Read the model definition and answer for the solid it produces. Units are mm, in the model's axes. A direction names the side the tool comes from. Give positions to 0.01 mm unless a question says otherwise; leave off trailing zeros. Loops run counter-clockwise (first coordinate to the right, second up) from the corner with the lowest first, then second, coordinate; pieces in that order, holes last.
(1) Which of the six approach directions +Z, -Z, +X, -X, +Y, -Y give full straight-line access (tool end or side, diameter ignored) to faces 4 (the face through (-2, 0, 0)), 5 (the face through (0, 0, 3)), 6 (the face through (2.44, -0.54, 5.8))?
(2) Find section B-B, the plane z = 9. Write down the section's boundary in (x, y), then the cut area to 3 significant figures.
(3) Determine the mould class of faces 1 (the face through (0, 0, 10)), 2 (the face through (5.37, -1.19, 1.01)), 3 (the face through (0.74, -1.305, 1.479)) for opening direction Y: pulls with the +Y half, pulls with the -Y half, needs draft (parallel to the pull), parting line crosses it, or undercut.
(4) Find section A-A, the plane y = 0. Write down the section's boundary in (x, z).
(5) Straight lines are drawn through the part: probe 1 along Z at (x, y) = (-3.5, -1.25); probe 2 along Y at (x, z) = (1, 1.5); probe 3 along Y at (x, z) = (0.25, 0.75). For each, find the intervals that lie inside material, in ascending order.
(6) Each of these flat-tipped pins is pushed along its axis until it touches: P1, Ø2, axis at x = -1.5, z = 7.5, coming from the -Y side; P2, Ø1.5, axis at x = -0.5, y = 0, coming from the -Z side; P3, Ø2, axis at y = 0.5, z = 7, coming from the -X side. Where does it stop, or does it pass through?
Autodesk Inventor part; units mm, degrees
ref_plane "YZ Plane" through (0, 0, 0) normal (1, 0, 0) x (0, 1, 0)
ref_plane "XZ Plane" through (0, 0, 0) normal (0, 1, 0) x (-1, 0, 0)
ref_plane "XY Plane" through (0, 0, 0) normal (0, 0, 1) x (1, 0, 0)
sketch "Sketch1" plane through (0, 0, 0) normal (1, 0, 0) x (0, 1, 0)
  line L0 (0, 0) -> (5.5, 0)
  line L1 (5.5, 0) -> (5.5, 2)
  line L2 (5.5, 2) -> (2.5, 2)
  line L3 (2.5, 2) -> (2.5, 10)
  line L4 (2.5, 10) -> (0, 10)
  line L5 (0, 10) -> (0, 0)
  dimension "d0" = 8
  dimension "d1" = 2
  dimension "d2" = 5.5
  dimension "d3" = 2.5
revolve "Revolution1" add sketch "Sketch1" angle 360 about axis through (0, 0, 10) along (0, 0, -1)
fillet "Fillet1" radius 0.5 3 edges at (0, -5.5, 0) (0, -5.5, 2) (0, -2.5, 10)
sketch "Sketch2" plane through (0, 0, 0) normal (0, 0, -1) x (-1, 0, 0)
  circle A0 centre (0, 0) radius 5
  line L0 (1.5, -0.866) -> (0, -1.7321)
  line L1 (0, -1.7321) -> (-1.5, -0.866)
  line L2 (-1.5, -0.866) -> (-1.5, 0.866)
  line L3 (-1.5, 0.866) -> (0, 1.7321)
  line L4 (0, 1.7321) -> (1.5, 0.866)
  line L5 (1.5, 0.866) -> (1.5, -0.866)
  dimension "d6" = 3
extrude "Extrusion1" cut sketch "Sketch2" against normal blind 3 contours L0 L1 L2 L3 L4 L5
thread "Thread1"
properties part number "M5x8 low profile screw"
Entries:
1. face 4: -Z, +X, -X, +Y, -Y
1. face 5: -Z
1. face 6: +Z
2. outline: circle Ø5 at (0, 0)
2. area: 19.6 mm2
3. face 1: needs draft
3. face 2: parting line crosses it
3. face 3: undercut
4. outline: (-5.5, 0.5) arc R0.5 ccw to (-5, 0) - (-1.5, 0) - (-1.5, 3) - (1.5, 3) - (1.5, 0) - (5, 0) arc R0.5 ccw to (5.5, 0.5) - (5.5, 1.5) arc R0.5 ccw to (5, 2) - (2.5, 2) - (2.5, 9.5) arc R0.5 ccw to (2, 10) - (-2, 10) arc R0.5 ccw to (-2.5, 9.5) - (-2.5, 2) - (-5, 2) arc R0.5 ccw to (-5.5, 1.5) - close
5. probe 1: z = 0 to 2
5. probe 2: y = -5.41 to -1.15, 1.15 to 5.41
5. probe 3: y = -5.49 to -1.59, 1.59 to 5.49
6. P1: stops at y = -2.45
6. P2: stops at z = 3
6. P3: stops at x = -2.5
